from build123d import *

# Parameters (mm, degrees)
SKIZZE2_R                        = 8
AUFSATZ_LINEAR_AUSTRAGEN1_DEPTH  = 4
F_3_0_3_DURCHMESSER_BOHRUNG1_D   = 3
SKIZZE8_R                        = 0.75
AUFSATZ_LINEAR_AUSTRAGEN2_DEPTH  = 2
F_1_5_1_5_DURCHMESSER_BOHRUNG1_D = 1.5
FASE1_SIZE                       = 0.5
FASE2_SIZE                       = 0.3
SKIZZE16_R                       = 0.75
SCHNITT_LINEAR_AUSTRAGEN1_DEPTH  = 5


with BuildPart() as part:
    # Skizze2 → Aufsatz-Linear austragen1 (new body)
    with BuildSketch(Plane.XY):
        Circle(SKIZZE2_R)
    extrude(amount=AUFSATZ_LINEAR_AUSTRAGEN1_DEPTH)

    # Ø3.0 (3) Durchmesser Bohrung1 (through all)
    with Locations(Plane(origin=(0, 0, 0), x_dir=(-1, 0, 0), z_dir=(0, 0, -1))):
        with Locations((0, 0)):
            Hole(F_3_0_3_DURCHMESSER_BOHRUNG1_D / 2)

    # Skizze9 → Schnitt-Rotation2 (revolve, cut)
    with BuildSketch(Plane(origin=(0, 0, 0), x_dir=(1, 0, 0), z_dir=(0, 1, 0))):
        with BuildLine():
            Line((-4.5, -2.5), (-8, -2.5))
            Line((-8, -2.5), (-8, -1))
            Line((-8, -1), (-4.5, -1))
            ThreePointArc((-4.5, -1), (-3.75, -1.75), (-4.5, -2.5))
        make_face()
    revolve(axis=Axis((0, 0, 0), (0, 0, 1)), mode=Mode.SUBTRACT)

    # Skizze8 → Aufsatz-Linear austragen2 (add)
    with BuildSketch(Plane.XY.offset(4)):
        with Locations((0, 6)):
            Circle(SKIZZE8_R)
        with Locations((6, 0)):
            Circle(SKIZZE8_R)
        with Locations((0, -6)):
            Circle(SKIZZE8_R)
        with Locations((-6, 0)):
            Circle(SKIZZE8_R)
    extrude(amount=AUFSATZ_LINEAR_AUSTRAGEN2_DEPTH)

    # Ø1.5 (1.5) Durchmesser Bohrung1 (through all)
    with Locations(Plane(origin=(0, 0, 0), x_dir=(1, 0, 0), z_dir=(0, 0, -1))):
        with Locations((-3.535533906, -3.535533906)):
            Hole(F_1_5_1_5_DURCHMESSER_BOHRUNG1_D / 2)

    # Fase1
    fase1_edges = [part.edges().sort_by_distance(p)[0] for p in [
        (-8, 0, 2.5),
        (-8, 0, 1),
    ]]
    chamfer(fase1_edges, length=FASE1_SIZE)

    # Fase2
    fase2_edges = [part.edges().sort_by_distance(p)[0] for p in [
        (-0.75, 6, 6),
        (5.25, 0, 6),
        (-0.75, -6, 6),
        (-6.75, 0, 6),
    ]]
    chamfer(fase2_edges, length=FASE2_SIZE)

    # Skizze16 → Schnitt-Linear austragen1 (cut)
    with BuildSketch(Plane.XY.offset(2)):
        with Locations((0, 6)):
            Circle(SKIZZE16_R)
        with Locations((6, 0)):
            Circle(SKIZZE16_R)
        with Locations((0, -6)):
            Circle(SKIZZE16_R)
        with Locations((-6, 0)):
            Circle(SKIZZE16_R)
    extrude(amount=SCHNITT_LINEAR_AUSTRAGEN1_DEPTH, mode=Mode.SUBTRACT)


solid = part.part
Can you work these out from the model? Positions are in its coordinate system, mm. A direction names the side the tool comes from. Give positions to 0.01 mm unless a question says otherwise; leave off trailing zeros. Loops run counter-clockwise (first coordinate to the right, second up) from the corner with the lowest first, then second, coordinate; pieces in that order, holes last. Notation, with made-up numbers: M 39.5,34.25 L 73.5,34.25 A11 cw 73.5,42.25 Z; hole C -3.75,-30 d7. An arc over 180 degrees is marked long. One line per item, written item: value. Start each with the question number.
1) If I drill on line 1 (Y direction, x = 0, z = 3.6); line 2 (Z direction, x = 1.25, y = -7); line 3 (Y direction, x = -1, z = 1.75), over which ranges is the centre line in solid material (lowest first)? Write a range as [from, to].
2) If we section it at C-C, the plane z = 3.6: Write out the boundary of the cut face in (x, y).
3) If we section it at D-D, the plane z = 1.55: Write out the boundary of the cut face in (x, y).
4) If we section it at A-A, the plane y = 0: Write out the boundary of the cut face in (x, z).
5) I'm going to push flat-ended pins straight in: pin 1 (0.9 mm diameter, centred on x = -6, y = 0, fed in from +Z); pin 2 (1.5 mm diameter, centred on x = 5, z = 3, fed in from -Y); pin 3 (1 mm diameter, centred on y = 2, z = 2.5, fed in from +X). Where does each tip first touch, or does it pass through?
6) On a 3-axis mill with a long thin cutter (end or side, diameter ignored), from which of +Z, -Z, +X, -X, +Y, -Y can I reach the whole of each face in a straight line? I mean faces 4 (the face through (-0.163, 5.268, 3.24)), 5 (the face through (-1.5, 0.07, 2.03)), 6 (the face through (3.4, 3.2, 1)). Say none if no direction works.
7) Thinking about a two-plate mould opening in X: for faces 1 (the face through (-3.939, 2.903, 3.239)), 2 (the face through (3.2, -3.4, 2.5)), 3 (the face through (-1.73, -7.81, 3.49)), which applies, +X half, -X half, draft (parallel to the pull), parting line (faces both ways), or undercut?
Completed:
1. line 1: y = [-8, -6.75], [-5.25, -1.5], [1.5, 5.25], [6.75, 8]
1. line 2: z = [0, 1], [2.5, 4]
1. line 3: y = [-3.61, -1.12], [1.12, 3.61]
2. outline: C 0,0 d16; hole C -6,0 d1.5; hole C -3.54,3.54 d1.5; hole C 0,0 d3; hole C 0,-6 d1.5; hole C 0,6 d1.5; hole C 6,0 d1.5
3. outline: C 0,0 d7.55; hole C 0,0 d3
4. outline: M -8,0 L -1.5,0 L -1.5,4 L -5.25,4 L -5.25,2.5 L -4.5,2.5 A0.75 cw -4.5,1 L -7.5,1 L -8,0.5 Z; M -8,3 L -7.5,2.5 L -6.75,2.5 L -6.75,4 L -8,4 Z; M 1.5,0 L 8,0 L 8,0.5 L 7.5,1 L 4.5,1 A0.75 cw 4.5,2.5 L 5.25,2.5 L 5.25,4 L 1.5,4 Z; M 6.75,2.5 L 7.5,2.5 L 8,3 L 8,4 L 6.75,4 Z
5. pin 1: stops at z = 1
5. pin 2: stops at y = -6.78
5. pin 3: stops at x = 7.76
6. face 4: +Z
6. face 5: +Z, -Z
6. face 6: none
7. face 1: undercut
7. face 2: draft
7. face 3: parting line
